CAD build for the part. Positions are in the model's coordinates, mm. Face numbers are marked on the shaded views. A direction names the side the tool comes from. Give positions to 0.01 mm unless a question says otherwise; leave off trailing zeros. Write each loop counter-clockwise with the first axis right and the second up, starting at its lowest first coordinate (ties: lowest second). Pieces come first, ordered by that corner, then holes. Notation, with made-up numbers: (-7.5, 13.25) - (17.5, 13.25) arc R9 cw to (17.5, 25.25) - close; hole circle Ø6 at (33.5, 34). An arc over 180 degrees is marked (long way). Answer as a JSON object with one key per item and string values.
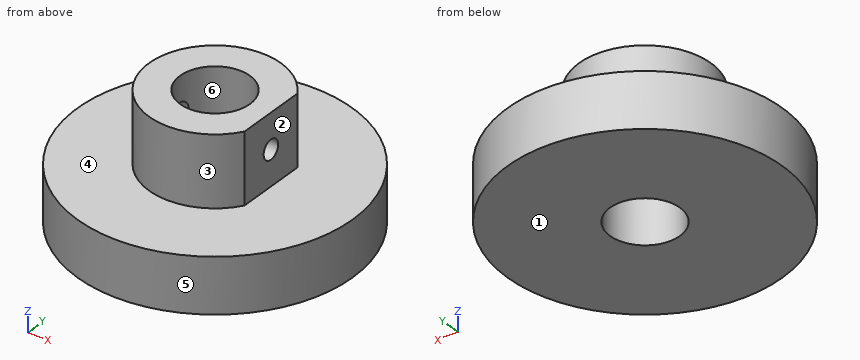
Autodesk Inventor part; units mm, degrees
ref_plane "YZ Plane" through (0, 0, 0) normal (1, 0, 0) x (0, 1, 0)
ref_plane "XZ Plane" through (0, 0, 0) normal (0, 1, 0) x (-1, 0, 0)
ref_plane "XY Plane" through (0, 0, 0) normal (0, 0, 1) x (1, 0, 0)
sketch "Sketch1" plane through (0, 0, 0) normal (0, 0, 1) x (1, 0, 0)
  circle A0 centre (0, 0) radius 25
  dimension "d0" = 50
extrude "Extrusion1" add sketch "Sketch1" along normal blind 10
sketch "Sketch14" plane through (0, 0, 10) normal (0, 0, 1) x (1, 0, 0)
  circle A0 centre (0, 0) radius 12
  line L0 (10.16, 0) -> (10.16, 6.3855)
  line L1 (10.16, -6.3855) -> (10.16, 0)
  dimension "d16" = 24
extrude "Extrusion4" add sketch "Sketch14" along normal blind 12.771 contours L0 L1 A0 picked at (-4.553, 0)
sketch "Sketch19" plane through (0, 0, 22.771) normal (0, 0, 1) x (1, 0, 0)
  circle A0 centre (0, 0) radius 6.35
  dimension "d28" = 12.7
extrude "Extrusion7" cut sketch "Sketch19" against normal blind 18
sketch "Sketch22" plane through (10.16, -6.3855, 10) normal (1, 0, 0) x (0, 0, -1)
  line L0 (-12.771, 0) -> (-12.771, 12.771)
  circle A0 centre (-6.3855, 6.3855) radius 1.75
  point P0 (10, 6.3855)
  dimension "d40" = 3.5
extrude "Extrusion10" cut sketch "Sketch22" against normal blind 25
sketch "Sketch23" plane through (0, 0, 4.771) normal (0, 0, 1) x (1, 0, 0)
  circle A0 centre (0, 0) radius 6.35
  dimension "d43" = 12.7
extrude "Extrusion11" cut sketch "Sketch23" against normal blind 10
equation "\"BendRadius\" = Thickness"
equation "\"BendReliefWidth\" = Thickness"
equation "\"BendReliefDepth\" = 0.5 * Thickness"
equation "\"CornerReliefSize\" = 4 * Thickness"
equation "\"MinimumRemnant\" = 2 * Thickness"
equation "\"TransitionRadius\" = BendRadius"
equation "\"JacobiRadiusSize\" = BendRadius"
equation "\"GapSize\" = Thickness"
properties part number "Project_Stationary_Wheel_Final"
Item 1: Probe line 1 (X direction, y = 0, z = 11); line 2 (Z direction, x = -1, y = 20); line 3 (X direction, y = 3, z = 18.5). List the from-to ranges inside material, lowest first. Write a range as from..to.
Entries:
{"line 1": "-12..-6.35, 6.35..10.16", "line 2": "0..10", "line 3": "-11.62..-5.6, 5.6..10.16"}
Item 2: Cut at B-B (x = 0). Give the cut face in (y, z), and give its area (3 significant figures).
Entries:
{"outline": "(-25, 0) - (-6.35, 0) - (-6.35, 22.77) - (-12, 22.77) - (-12, 10) - (-25, 10) - close; (6.35, 0) - (25, 0) - (25, 10) - (12, 10) - (12, 22.77) - (6.35, 22.77) - close", "area": "517 mm2"}
Item 3: Flat gauge pins, fed straight in: P1, Ø1.5, axis at x = 1, y = 19.5, coming from the +Z side; P2, Ø10, axis at y = -10, z = 7, coming from the +X side; P3, Ø4, axis at y = 2.5, z = 13.5, coming from the +X side. Where does each tip first touch, or does it go through?
Entries:
{"P1": "z = 10", "P2": "x = 24.49", "P3": "x = 10.16"}
Item 4: Cut at D-D (z = 17.25). Give the cut face in (x, y).
Entries:
{"outline": "(-11.9, -1.52) arc R12 ccw to (10.16, -6.39) - (10.16, -1.52) - (6.17, -1.52) arc R6.35 cw to (-6.17, -1.52) - close; (-11.9, 1.52) - (-6.17, 1.52) arc R6.35 cw to (6.17, 1.52) - (10.16, 1.52) - (10.16, 6.39) arc R12 ccw to start"}
Item 5: Mould opens along X. For the marked faces 4, 5 and 6 say: +X half, -X half, draft (parallel to the pull), parting line (faces both ways), or undercut.
Entries:
{"face 4": "draft", "face 5": "parting line", "face 6": "undercut"}
Item 6: Cut at C-C (z = 8). Give the cut face in (x, y).
Entries:
{"outline": "circle Ø50 at (0, 0); hole circle Ø12.7 at (0, 0)"}
Item 7: Cut at A-A (y = 0). Give the cut face in (x, z), and give its area (3 significant figures).
Entries:
{"outline": "(-25, 0) - (-6.35, 0) - (-6.35, 14.64) - (-12, 14.64) - (-12, 10) - (-25, 10) - close; (-12, 18.14) - (-6.35, 18.14) - (-6.35, 22.77) - (-12, 22.77) - close; (6.35, 0) - (25, 0) - (25, 10) - (10.16, 10) - (10.16, 14.64) - (6.35, 14.64) - close; (6.35, 18.14) - (10.16, 18.14) - (10.16, 22.77) - (6.35, 22.77) - close", "area": "461 mm2"}
Item 8: Which spindle directions (+Z, -Z, +X, -X, +Y, -Y) get a long thin tool onto all of the face, cutting with end or side? Do the marked faces 1, 2 and 3. Say none if no direction does.
Entries:
{"face 1": "-Z, +X, -X, +Y, -Y", "face 2": "+Z, +X, +Y, -Y", "face 3": "+Z"}
